Read the model definition and answer for the solid it produces. Units are mm, in the model's axes. Round coordinates to 2 decimals unless told otherwise and drop trailing zeros. Use one line per item in the form item = value. Start each with the question number.
from build123d import *

# Parameters (mm, degrees)
BOSS_EXTRUDE1_DEPTH = 45
REVOLVE1_ANGLE      = 180
BOSS_EXTRUDE2_DEPTH = 15


with BuildPart() as part:
    # Sketch1 → Boss-Extrude1 (new body)
    with BuildSketch(Plane.XY):
        with BuildLine():
            Line((0, 0), (37.46998799, 0))
            ThreePointArc((37.46998799, 0), (18.734993995, 27), (0, 0))
        make_face()
    extrude(amount=BOSS_EXTRUDE1_DEPTH)



with BuildPart() as body_2:
    # Sketch4 → Revolve1 (revolve)
    with BuildSketch(Plane.XY.offset(60)):
        with BuildLine():
            Line((18.734993995, 0), (18.734993995, 39.259436234))
            add(Edge.make_bspline(
                [(18.734993995, 39.259436234), (46.178787864, 39.232586668), (48.009362148, 8.206101436), (37.46998799, 0)],
                knots=[0, 0, 0, 0, 1, 1, 1, 1], degree=3))
            Line((37.46998799, 0), (18.734993995, 0))
        make_face()
    revolve(axis=Axis((18.734993995, 0, 60), (0, 1, 0)), revolution_arc=REVOLVE1_ANGLE)


with BuildPart() as part_1:
    add(part.part)

    add(body_2.part)  # Boss-Extrude2 merges body 2
    # Sketch5 → Boss-Extrude2 (add)
    with BuildSketch(Plane.XY.offset(45)):
        with BuildLine():
            Line((0, 0), (37.46998799, 0))
            ThreePointArc((37.46998799, 0), (18.734993995, 27), (0, 0))
        make_face()
    extrude(amount=BOSS_EXTRUDE2_DEPTH)


solid = part_1.part
Item 1: For a pull along Z with two mould halves and no side action, classify faces 1 (the flat face through (18, 0, 30)), 2 (the flat face through (19, 20, 60)), 3 (the flat face through (18, 11, 0)) as pulls with the +Z half, pulls with the -Z half, needs draft (parallel to the pull), parting line crosses it, or undercut.
Item 2: Given P1, Ø10, axis at y = 24.5, z = 34, coming from the -X side; P2, Ø2, axis at y = 26.5, z = 27, coming from the +X side; P3, Ø5, axis at x = 9, z = 23, coming from the +Y side, each flat-ended and moving along its own axis, determine where each tip first touches the part or whether it passes through.
Item 3: Find the intervals of material crossed by L1, parallel to Y at x = 6.5, z = 32.5; L2, parallel to Y at x = 9, z = 18; L3, parallel to X at y = 8.5, z = 13, in increasing order. Write a range as [from, to].
The answers:
q1.face_1 = needs draft
q1.face_2 = pulls with the +Z half
q1.face_3 = pulls with the -Z half
q2.P1 = 3.12
q2.P2 = 26.33
q2.P3 = 25.65
q3.L1 = [0, 22.82]
q3.L2 = [0, 24.47]
q3.L3 = [-1.21, 38.68]
